Input: part model. Units: mm. Frame: model coordinates. Face numbers are marked on the shaded views. A direction names the side the tool comes from. Give positions to 0.01 mm unless a question says otherwise; leave off trailing zeros. Order: outer loops, then holes, each group sorted by start corner. A loop starts at its lowest first (then second) coordinate and runs counter-clockwise, first axis right, second up. Notation, with made-up numbers: (23, 44) - (81, 44) arc R18 ccw to (81, 54) - close; hole circle Ø10 at (79.25, 78). An arc over 180 degrees is marked (long way). Answer in a Markdown table with one row per item. Add a question column.
1. Access query for the marked faces 4, 5 and 6. Directions: +Z, -Z, +X, -X, +Y, -Y. A direction counts if a zero-diameter tool reaches every point of the face in a straight line with its end or side. Return the directions, or none.
2. Section query A-A on x = -2.25. Return loops of the section in (y, z), and give its area (3 significant figures).
3. Ray query, line 1 (Y direction, x = 0.25, z = 0); line 2 (X direction, y = 2, z = 2.5); line 3 (X direction, y = -2.75, z = 0.25). Return the intervals inside material, ascending. Write a range as [from, to].
4. Mould query, pull axis Z, two halves, no side actions, for the marked faces 1, 2 and 3. Classes: released by +Z, released by -Z, zero draft, split by the parting line, or undercut.
5. Contact query for flat-ended pins moving along their axis: pin 1 (3 mm diameter, centred on y = 1, z = 1, fed in from -X); pin 2 (1 mm diameter, centred on x = -1, z = 1, fed in from -Y); pin 3 (2 mm diameter, centred on y = 2, z = -1.5, fed in from -X); pin 4 (1 mm diameter, centred on x = 3.5, y = 2.5, fed in from +Z). Output: stop coordinate, or through.
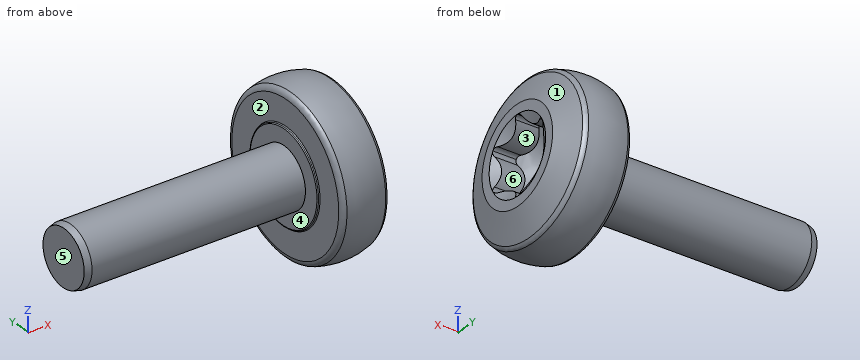
```python
from build123d import *

# Parameters (mm, degrees)
BOSS_EXTRUDE1_REACH = 14.932
SKETCH3_R           = 2.0335875
FILLET1_R           = 0.24638
CHAMFER1_SIZE       = 0.280736842
CHAMFER1_SIZE2      = 0.07522321


with BuildPart() as part:
    # Sketch2 → Revolve1 (revolve)
    with BuildSketch(Plane.XY, mode=Mode.PRIVATE) as revolve1_sk:
        with BuildLine():
            Line((-5.9944, 0), (5.9944, 0))
            Line((5.9944, 0), (5.9944, 2.0335875))
            Line((5.9944, 2.0335875), (5.50164, 3.25755))
            ThreePointArc((5.50164, 3.25755), (4.51612, 3.429), (3.5306, 3.25755))
            Line((3.5306, 3.25755), (3.5306, 2.003369298))
            ThreePointArc((3.5306, 2.003369298), (3.519440768, 1.97642853), (3.4925, 1.965269298))
            ThreePointArc((3.4925, 1.965269298), (3.465559232, 1.954110067), (3.4544, 1.927169298))
            Line((3.4544, 1.927169298), (3.4544, 1.261978947))
            Line((3.4544, 1.261978947), (-5.9944, 1.261978947))
            Line((-5.9944, 1.261978947), (-5.9944, 0))
        make_face()
    revolve(revolve1_sk.sketch.rotate(Axis((-5.9944, 0, 0), (-1, 0, 0)), 90), axis=Axis((-5.9944, 0, 0), (-1, 0, 0)))

    # Sketch12 → Cut-Revolve3 (revolve, cut)
    with BuildSketch(Plane.XY, mode=Mode.PRIVATE) as cut_revolve3_sk:
        Polygon((5.9944, 1.6256), (4.99348125, 1.6256), (4.054940652, 0), (5.9944, 0), align=None)
    revolve(cut_revolve3_sk.sketch.rotate(Axis((-5.9944, 0, 0), (1, 0, 0)), 270), axis=Axis((-5.9944, 0, 0), (1, 0, 0)), mode=Mode.SUBTRACT)

    # Boss-Extrude1: up to this cone (the profile starts inside it)
    boss_extrude1_end = Plane(origin=(5.9944, 0, 0), z_dir=(1, 0, 0)).offset(-1.939458348) * Cone(1.732e-06, 35.906628234, 20.730700477, align=(Align.CENTER, Align.CENTER, Align.MIN), mode=Mode.PRIVATE)
    # Sketch3 → Boss-Extrude1 (add, up to the surface)
    with BuildSketch(Plane(origin=(5.9944, 0, 0), x_dir=(0, 0, -1), z_dir=(1, 0, 0)), mode=Mode.PRIVATE) as boss_extrude1_sk1:
        Circle(SKETCH3_R)
        with BuildLine():
            ThreePointArc((1.51222877, -0.182266377), (1.594944844, -0.107324354), (1.6256, 0))
            ThreePointArc((1.6256, 0), (1.594944844, 0.107324354), (1.51222877, 0.182266377))
            ThreePointArc((1.51222877, 0.182266377), (1.055858172, 0.6096), (0.913961698, 1.218495343))
            ThreePointArc((0.913961698, 1.218495343), (0.890418039, 1.327600575), (0.8128, 1.407810896))
            ThreePointArc((0.8128, 1.407810896), (0.704526805, 1.434924929), (0.598267073, 1.40076172))
            ThreePointArc((0.598267073, 1.40076172), (0, 1.2192), (-0.598267073, 1.40076172))
            ThreePointArc((-0.598267073, 1.40076172), (-0.704526805, 1.434924929), (-0.8128, 1.407810896))
            ThreePointArc((-0.8128, 1.407810896), (-0.890418039, 1.327600575), (-0.913961698, 1.218495343))
            ThreePointArc((-0.913961698, 1.218495343), (-1.055858172, 0.6096), (-1.51222877, 0.182266377))
            ThreePointArc((-1.51222877, 0.182266377), (-1.594944844, 0.107324354), (-1.6256, 0))
            ThreePointArc((-1.6256, 0), (-1.594944844, -0.107324354), (-1.51222877, -0.182266377))
            ThreePointArc((-1.51222877, -0.182266377), (-1.055858172, -0.6096), (-0.913961698, -1.218495343))
            ThreePointArc((-0.913961698, -1.218495343), (-0.890418039, -1.327600575), (-0.8128, -1.407810896))
            ThreePointArc((-0.8128, -1.407810896), (-0.704526805, -1.434924929), (-0.598267073, -1.40076172))
            ThreePointArc((-0.598267073, -1.40076172), (0, -1.2192), (0.598267073, -1.40076172))
            ThreePointArc((0.598267073, -1.40076172), (0.704526805, -1.434924929), (0.8128, -1.407810896))
            ThreePointArc((0.8128, -1.407810896), (0.890418039, -1.327600575), (0.913961698, -1.218495343))
            ThreePointArc((0.913961698, -1.218495343), (1.055858172, -0.6096), (1.51222877, -0.182266377))
        make_face(mode=Mode.SUBTRACT)
    boss_extrude1_tool1 = extrude(boss_extrude1_sk1.sketch, amount=-BOSS_EXTRUDE1_REACH, mode=Mode.PRIVATE) & boss_extrude1_end
    add(boss_extrude1_tool1.solids().sort_by_distance((5.9944, 0, 1.976069))[0])

    # Cut-Extrude2 cone 1 section (on through the dimple's axis) → Cut-Extrude2 (revolve, cut)
    with BuildSketch(Plane(origin=(5.9944, 0, 0), x_dir=(0, 0, -1), z_dir=(0, 1, 0))):
        Polygon((0, 0), (1.6256, 0), (0, 0.938540598), align=None)
    revolve(axis=Axis((5.9944, 0, 0), (-1, 0, 0)), mode=Mode.SUBTRACT)

    # Fillet1
    fillet1_edges = [part.edges().sort_by_distance(p)[0] for p in [
        (3.5306, 0, 3.25755),
        (5.50164, 0, 3.25755),
    ]]
    fillet(fillet1_edges, radius=FILLET1_R)

    # Chamfer1
    chamfer1_edges = [part.edges().sort_by_distance(p)[0] for p in [
        (-5.9944, 0, 1.261978947),
    ]]
    chamfer1_side = [part.faces().sort_by_distance(p)[0] for p in [
        (-1.27, 0, 1.261978947),
    ]]
    chamfer(chamfer1_edges, length=CHAMFER1_SIZE, length2=CHAMFER1_SIZE2, reference=chamfer1_side[0])


solid = part.part
```
Answer:
| question | item | result |
|---|---|---|
| 1 | face 4 | -X |
| 1 | face 5 | +Z, -Z, -X, +Y, -Y |
| 1 | face 6 | +X |
| 2 | outline | circle Ø2.52 at (0, 0) |
| 2 | area | 5.00 mm² |
| 3 | line 1 | y = [-1.26, 1.26] |
| 3 | line 2 | x = [3.56, 5.52] |
| 3 | line 3 | x = [3.53, 5.7] |
| 4 | face 1 | split by the parting line |
| 4 | face 2 | zero draft |
| 4 | face 3 | undercut |
| 5 | pin 1 | stops at x = -5.99 |
| 5 | pin 2 | stops at y = -1.16 |
| 5 | pin 3 | stops at x = 3.45 |
| 5 | pin 4 | stops at z = 2.61 |
